The drawing under review shows one solid part. Ordinate dimensions are in mm from its lowest x, y, z. A direction names the side the tool comes from. Coordinates: 2 decimals unless noted, no trailing zeros. Write each loop counter-clockwise with the first axis right and the second up, starting at its lowest first coordinate (ties: lowest second). Pieces come first, ordered by that corner, then holes.
1) Add section A-A, the plane x = 3.81. State the section outline as (y, z) points, then the cut area to 3 significant figures.
2) Add section D-D, the plane y = 13.97. State the section outline as (x, z) points, then the cut area to 3 significant figures.
3) Machinability: for the marked faces 4, 5 and 6, which of the approach directions +Z, -Z, +X, -X, +Y, -Y give a long, thin tool a straight path to every point of the face, cutting with its end or side? Answer none if there is none.
4) Add section C-C, the plane z = 15. State the section outline as (x, y) points, then the cut area to 3 significant figures.
5) For P1, Ø6.5, axis at x = 10.5, z = 15.5, coming from the -Y side; P2, Ø5, axis at x = 10, z = 16, coming from the +Y side; P3, Ø3, axis at y = 13.42, z = 8.26, coming from the +X side; P4, Ø4, axis at x = 13.5, y = 17.5, coming from the -Z side, all flat-tipped, find the tip position at first contact; note any pin that passes through.
6) Mouldability with a two-part tool opening along X and no side actions: class the marked faces 1, 2 and 3 as released by +X, released by -X, zero draft, split by the parting line, or undercut.
7) Add section B-B, the plane y = 3.81. State the section outline as (x, z) points, then the cut area to 3 significant figures.
8) For line 1 (Y direction, x = 16.5, z = 18.5); line 2 (Z direction, x = 16.25, y = 10); line 3 (X direction, y = 8.75, z = 11.75), list the stretches that pass through material, from the lowest coordinate up.
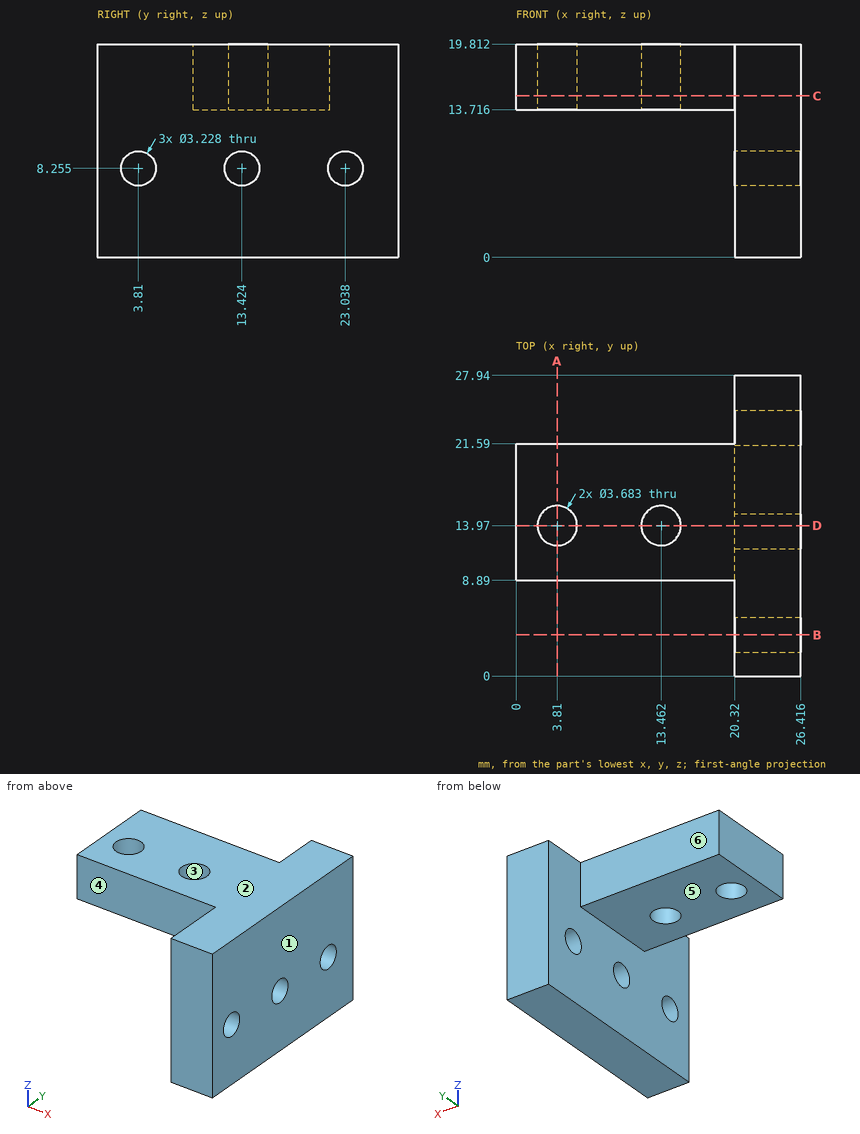
Geometry results:
1. outline: (8.89, 13.72) - (12.13, 13.72) - (12.13, 19.81) - (8.89, 19.81) - close; (15.81, 13.72) - (21.59, 13.72) - (21.59, 19.81) - (15.81, 19.81) - close
1. area: 55.0 mm2
2. outline: (0, 13.72) - (1.97, 13.72) - (1.97, 19.81) - (0, 19.81) - close; (5.65, 13.72) - (11.62, 13.72) - (11.62, 19.81) - (5.65, 19.81) - close; (15.3, 13.72) - (20.32, 13.72) - (20.32, 9.77) - (26.42, 9.77) - (26.42, 19.81) - (15.3, 19.81) - close; (20.32, 0) - (26.42, 0) - (26.42, 6.74) - (20.32, 6.74) - close
2. area: 181 mm2
3. face 4: +Z, -Z, -X, -Y
3. face 5: -Z, -X, +Y, -Y
3. face 6: +Z, -Z, -X, +Y
4. outline: (0, 8.89) - (20.32, 8.89) - (20.32, 0) - (26.42, 0) - (26.42, 27.94) - (20.32, 27.94) - (20.32, 21.59) - (0, 21.59) - close; hole circle Ø3.68 at (3.81, 13.97); hole circle Ø3.68 at (13.46, 13.97)
4. area: 407 mm2
5. P1: stops at y = 8.89
5. P2: stops at y = 21.59
5. P3: passes through
5. P4: stops at z = 13.72
6. face 1: released by +X
6. face 2: zero draft
6. face 3: undercut
7. outline: (20.32, 0) - (26.42, 0) - (26.42, 6.64) - (20.32, 6.64) - close; (20.32, 9.87) - (26.42, 9.87) - (26.42, 19.81) - (20.32, 19.81) - close
7. area: 101 mm2
8. line 1: y = 8.89 to 21.59
8. line 2: z = 13.72 to 19.81
8. line 3: x = 20.32 to 26.42
